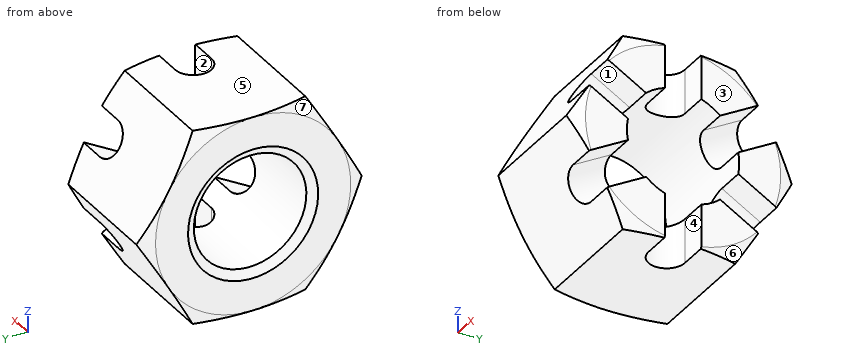
Autodesk Inventor part; units mm, degrees
ref_plane "Work Plane1" through (18.75, 0, 0) normal (0, -0.5, -0.866) x (0, -0.866, 0.5)
ref_plane "YZ Plane" through (0, 0, 0) normal (1, 0, 0) x (0, 1, 0)
ref_plane "XZ Plane" through (0, 0, 0) normal (0, 1, 0) x (-1, 0, 0)
sketch "Sketch1" plane through (0, 0, 0) normal (1, 0, 0) x (0, 1, 0)
  line L0 (-10.3923, 18) -> (10.3923, 18)
  line L1 (10.3923, 18) -> (20.7846, 0)
  line L2 (20.7846, 0) -> (10.3923, -18)
  line L3 (10.3923, -18) -> (-10.3923, -18)
  line L4 (-10.3923, -18) -> (-20.7846, 0)
  line L5 (-20.7846, 0) -> (-10.3923, 18)
  point P0 (0, 0)
  point P1 (0, 0)
  dimension "d0" = 41.5692
extrude "Body" add sketch "Sketch1" along normal blind 23.9
sketch "Sketch2" plane through (0, 0, 0) normal (0, 0, 1) x (1, 0, 0)
  line L0 (0, 10.3923) -> (0, 20.7846)
  line L1 (0, 20.7846) -> (23.9, 20.7846)
  line L2 (23.9, 10.3923) -> (23.9, 20.7846)
  line L3 (-4.78, 0) -> (28.68, 0)
  line L4 (1.2985, 20.7846) -> (0, 18)
  line L5 (22.6015, 20.7846) -> (23.9, 18)
  dimension "d3" = 25
  dimension "d4" = 25
  dimension "d5" = 36
  dimension "d6" = 36
revolve "Chamfer1" cut sketch "Sketch2" angle 360 about axis through (-10, 0, 0) along (1, 0, 0)
sketch "Sketch3" plane through (0, 0, 0) normal (0, 0, 1) x (1, 0, 0)
  line L0 (23.9, 0) -> (23.9, 15.5885)
  line L1 (23.9, -15.5885) -> (23.9, 0)
  line L2 (0, 15.5885) -> (0, 0)
  line L3 (0, 0) -> (0, -15.5885)
  line L4 (-4.78, 0) -> (28.68, 0)
  arc A0 (18.75, 3.35) -> (18.75, -3.35) centre (18.75, 0) ccw
  line L5 (18.75, 3.35) -> (23.9, 3.35)
  line L6 (18.75, -3.35) -> (23.9, -3.35)
  line L7 (23.9, -15.5885) -> (23.9, 0)
  dimension "d8" = 15.4
  dimension "d9" = 6.7
extrude "Groove" cut sketch "Sketch3" along normal through all
pattern_circular "Grooves" count 6 over 360 about axis through (-10, 0, 0) along (1, 0, 0) of "Groove"
sketch "Sketch4" plane through (0, 0, 0) normal (-1, 0, 0) x (0, 0, 1)
  arc A0 (-9, -15.5885) -> (9, -15.5885) centre (0, 0) ccw
hole "Thread" at (0, 0, 0) direction (1, 0, 0) diameter 20.752 end through all
chamfer "Chamfer2" distance 1.6238 angle 30 1 edges at (0, 0, -10.376) measured on face at (0, -15.3677, 0.4169)
ref_plane "Work Plane1" through (18.75, 0, 0) normal (0, -0.5, -0.866) x (0, -0.866, 0.5)
equation "\"d0\" = 1.1547 * SW"
equation "\"d1\" = KOH"
equation "\"d3\" = ANG1"
equation "\"d4\" = ANG2"
equation "\"d5\" = SW0"
equation "\"d6\" = SW01"
equation "\"d8\" = KOH1"
equation "\"d9\" = SNB"
equation "\"d11\" = KOH"
equation "\"d15\" = -0.5 * GD1 + 0.5 * NND"
equation "\"d35\" = -0.5 * GD1 + 0.5 * NND"
equation "\"ANG1\" = 25deg"
equation "\"ANG2\" = 25deg"
equation "\"NND\" = 24"
equation "\"KOH\" = 23.9"
equation "\"SW\" = 36"
equation "\"SNB\" = 6.7"
equation "\"KOH1\" = 15.4"
equation "\"SW01\" = SW"
equation "\"SW0\" = SW"
equation "\"d37\" = KOH1 - 0.288675 * NND + 0.288675 * GD1"
equation "\"GUL\" = 0.541266 * PTC"
equation "\"THREADDIA\" = 24"
equation "\"TOA\" = 30deg"
equation "\"PTC\" = 3"
equation "\"E0\" = 1.155 * SW"
equation "\"GAL\" = 0.541266 * PTC"
properties part number "ANSI B18.2.4.3M - M24 x 3" material "Steel, Mild"
CAD build for the part. Positions are in the model's coordinates, mm. Face numbers are marked on the shaded views. A direction names the side the tool comes from. Give positions to 0.01 mm unless a question says otherwise; leave off trailing zeros. Write each loop counter-clockwise with the first axis right and the second up, starting at its lowest first coordinate (ties: lowest second). Pieces come first, ordered by that corner, then holes. Notation, with made-up numbers: M 1.25,25 L 15.25,25 A26 ccw 15.25,49 Z; hole C 51,-37 d6. An arc over 180 degrees is marked long. Return JSON: item names as keys, results as strings. Group by question number.
(1) Flat gauge pins, fed straight in: pin 1 Ø4 at (x, z) = (17, 13) entering from -Y; pin 2 Ø4 at (x, z) = (20, -12.5) entering from -Y; pin 3 Ø8 at (x, z) = (12.5, 5.5) entering from +Y. Where does each tip first touch, or does it go through?
(2) 3-axis set-ups, long thin cutter, end or side, ignore diameter. For the marked faces 1, 2 and 3: which of +Z, -Z, +X, -X, +Y, -Y reach the whole face in a straight line?
(3) Drill centre lines: L1, parallel to Z at x = 11.75, y = 0; L2, parallel to Y at x = 18.75, z = 0; L3, parallel to Z at x = 20.25, y = -13.5. Where is each one in solid material? Low to high. Write a range as [from, to].
(4) Band-saw the part on A-A (x = 14). Give the cut face in (y, z), and give its area (3 significant figures).
(5) Mould opens along Y. For the marked faces 4, 5, 6 and 7 say: pulls with the +Y half, pulls with the -Y half, needs draft (parallel to the pull), parting line crosses it, or undercut.
Entries:
{
 "1": {"pin 1": "stops at y = -14.38", "pin 2": "stops at y = -13.94", "pin 3": "stops at y = 19.92"},
 "2": {"face 1": "+X, -Y", "face 2": "+Z, -Z, +X", "face 3": "+Z, -Z, +X, +Y, -Y"},
 "3": {"L1": "z = [-18, -10.38], [10.38, 18]", "L2": "y = [-20.78, -10.38], [10.38, 20.78]", "L3": "z = [-12.62, -11.66], [-3.93, 3.93], [11.66, 12.62]"},
 "4": {"outline": "M -20.78,0 L -10.39,-18 L 10.39,-18 L 20.78,0 L 10.39,18 L -10.39,18 Z; hole C 0,0 d20.75", "area": "784 mm^2"},
 "5": {"face 4": "undercut", "face 5": "needs draft", "face 6": "pulls with the +Y half", "face 7": "pulls with the -Y half"}
}
